Build history of the part. All positions in model axes, mm. A direction names the side the tool comes from. Round coordinates to 2 decimals unless told otherwise and drop trailing zeros. Write each loop counter-clockwise with the first axis right and the second up, starting at its lowest first coordinate (ties: lowest second). Pieces come first, ordered by that corner, then holes. Notation, with made-up numbers: (51.5, -31) -> (99.5, -31) arc R4 cw to (99.5, -26) -> close; hole circle Ø8 at (72, -36). An arc over 180 degrees is marked (long way). Answer as CSV lines item,"result".
from build123d import *

# Parameters (mm, degrees)
SKETCH_1_W          = 250
SKETCH_1_H          = 125
EXTRUDE_1_DEPTH     = 60.8
SKETCH_4_W          = 250
SKETCH_4_H          = 125
EXTRUDE_2_DEPTH     = 6
EXTRUDE_2_TAPER     = 35
SKETCH_5_W          = 241.597509542
SKETCH_5_H          = 116.597509542
EXTRUDE_3_DEPTH     = 12
SHELL_1_T           = -1.2
SKETCH_9_R          = 13
CUT_EXTRUDE_2_DEPTH = 12
SKETCH_10_R         = 13
CUT_EXTRUDE_3_DEPTH = 12


with BuildPart() as part:
    # 草图1 → 凸台-拉伸1 (new body)
    with BuildSketch(Plane.XY):
        Rectangle(SKETCH_1_W, SKETCH_1_H)
    extrude(amount=EXTRUDE_1_DEPTH)

    # 草图4 → 凸台-拉伸2 (add)
    with BuildSketch(Plane.XY.offset(60.8)):
        Rectangle(SKETCH_4_W, SKETCH_4_H)
    extrude(amount=EXTRUDE_2_DEPTH, taper=EXTRUDE_2_TAPER)

    # 草图5 → 凸台-拉伸3 (add)
    with BuildSketch(Plane.XY.offset(66.8)):
        Rectangle(SKETCH_5_W, SKETCH_5_H)
    extrude(amount=EXTRUDE_3_DEPTH)

    # 抽壳1
    shell_1_openings = [part.faces().sort_by_distance(p)[0] for p in [
        (0, 0, 78.8),
    ]]
    offset(amount=SHELL_1_T, openings=shell_1_openings, kind=Kind.INTERSECTION)

    # 草图9 → 切除-拉伸2 (cut)
    with BuildSketch(Plane.ZY.offset(125)):
        with Locations((35, 0)):
            Circle(SKETCH_9_R)
    extrude(amount=-CUT_EXTRUDE_2_DEPTH, mode=Mode.SUBTRACT)

    # 草图10 → 切除-拉伸3 (cut)
    with BuildSketch(Plane(origin=(125, 0, 0), x_dir=(0, 0, -1), z_dir=(1, 0, 0))):
        with Locations((-35, 31.25)):
            Circle(SKETCH_10_R)
        with Locations((-35, -31.25)):
            Circle(SKETCH_10_R)
    extrude(amount=-CUT_EXTRUDE_3_DEPTH, mode=Mode.SUBTRACT)


solid = part.part
1. Cut at B-B, the plane z = 35. Write the cut outline in (x, y), then the cut area to 3 significant figures.
Results found:
outline,"(-125, -62.5) -> (125, -62.5) -> (125, -44.25) -> (123.8, -44.25) -> (123.8, -61.3) -> (-123.8, -61.3) -> (-123.8, -13) -> (-125, -13) -> close; (-125, 13) -> (-123.8, 13) -> (-123.8, 61.3) -> (123.8, 61.3) -> (123.8, 44.25) -> (125, 44.25) -> (125, 62.5) -> (-125, 62.5) -> close; (123.8, -18.25) -> (125, -18.25) -> (125, 18.25) -> (123.8, 18.25) -> close"
area,"801 mm2"
2. Drop flat-ended pins along their axis: pin 1 Ø6 at (y, z) = (3.5, 75) entering from +X; pin 2 Ø23.5 at (y, z) = (31.25, 35) entering from +X; pin 3 Ø6 at (y, z) = (2.5, 70.5) entering from -X. Give the stop position or say it passes through.
Results found:
pin 1,"stops at x = 120.8"
pin 2,"stops at x = -123.8"
pin 3,"stops at x = -120.8"
3. Mould opens along Y. For faces 1 (the flat face through (121.73, 0.86, 63.38)), 2 (the flat face through (120.799, -1, 73)), 3 (the flat face through (1.8, -60.4, 63.8)) say: +Y half, -Y half, draft (parallel to the pull), parting line (faces both ways), or undercut.
Results found:
face 1,"undercut"
face 2,"draft"
face 3,"-Y half"
4. Cut at D-D, the plane z = 16.5. Write the cut outline in (x, y), then the cut area to 3 significant figures.
Results found:
outline,"(-125, -62.5) -> (125, -62.5) -> (125, 62.5) -> (-125, 62.5) -> close; hole (-123.8, -61.3) -> (123.8, -61.3) -> (123.8, 61.3) -> (-123.8, 61.3) -> close"
area,"894 mm2"
5. Cut at A-A, the plane y = 0. Write the cut outline in (x, z), then the cut area to 3 significant figures.
Results found:
outline,"(-125, 0) -> (125, 0) -> (125, 60.8) -> (120.8, 66.8) -> (120.8, 78.8) -> (119.6, 78.8) -> (119.6, 66.42) -> (123.8, 60.42) -> (123.8, 1.2) -> (-123.8, 1.2) -> (-123.8, 22) -> (-125, 22) -> close; (-125, 48) -> (-123.8, 48) -> (-123.8, 60.42) -> (-119.6, 66.42) -> (-119.6, 78.8) -> (-120.8, 78.8) -> (-120.8, 66.8) -> (-125, 60.8) -> close"
area,"458 mm2"
6. Probe line 1 along Y through (x, z) = (124.4, 35); line 2 along Y through (x, z) = (-16, 67.5); line 3 along X through (y, z) = (-47, 58.5). List the from-to ranges inside material, lowest first.
Results found:
line 1,"y = -62.5 to -44.25, -18.25 to 18.25, 44.25 to 62.5"
line 2,"y = -58.3 to -57.1, 57.1 to 58.3"
line 3,"x = -125 to -123.8, 123.8 to 125"
7. Cut at C-C, the plane x = -87. Write the cut outline in (y, z), then the cut area to 3 significant figures.
Results found:
outline,"(-62.5, 0) -> (62.5, 0) -> (62.5, 60.8) -> (58.3, 66.8) -> (58.3, 78.8) -> (57.1, 78.8) -> (57.1, 66.42) -> (61.3, 60.42) -> (61.3, 1.2) -> (-61.3, 1.2) -> (-61.3, 60.42) -> (-57.1, 66.42) -> (-57.1, 78.8) -> (-58.3, 78.8) -> (-58.3, 66.8) -> (-62.5, 60.8) -> close"
area,"339 mm2"
8. Which spindle directions (+Z, -Z, +X, -X, +Y, -Y) get a long thin tool onto all of the face, cutting with end or side? Do faces 4 (the cylindrical face through (-124.408, 0.572, 22.013)), 5 (the flat face through (119.599, -1, 73)), 6 (the flat face through (-2, -62.5, 30)), 7 (the flat face through (123.8, -1, 30)), 8 (the cylindrical face through (124.41, -22.46, 44.58)). Say none if no direction does.
Results found:
face 4,"-X"
face 5,"+Z"
face 6,"+Z, -Z, +X, -X, -Y"
face 7,"none"
face 8,"+X"
